CAD build for the part. Positions are in the model's coordinates, mm. A direction names the side the tool comes from. Give positions to 0.01 mm unless a question says otherwise; leave off trailing zeros. Write each loop counter-clockwise with the first axis right and the second up, starting at its lowest first coordinate (ties: lowest second). Pieces come first, ordered by that corner, then holes. Notation, with made-up numbers: (-31, 47) - (8, 47) arc R16 ccw to (8, 68) - close; hole circle Ø11 at (51, 38.25). An arc over 180 degrees is marked (long way). Write item = value, one per line. Start each with the question number.
```python
from build123d import *

# Parameters (mm, degrees)
ESQUISSE1_R             = 6
BOSS_EXTRU_1_DEPTH      = 10
ESQUISSE4_R             = 4.25
ESQUISSE4_R_2           = 3.25
ENL_V_MAT_EXTRU_1_DEPTH = 0.1


with BuildPart() as part:
    # Esquisse1 → Boss.-Extru.1 (new body)
    with BuildSketch(Plane(origin=(0, 0, 0), x_dir=(1, 0, 0), z_dir=(0, 1, 0))):
        with Locations(Location((0, 0, 0), (0, 0, 270))):
            Circle(ESQUISSE1_R)
    extrude(amount=-BOSS_EXTRU_1_DEPTH)

    # Esquisse3 → Révolution1 (revolve)
    with BuildSketch(Plane(origin=(0, 0, 0), x_dir=(0, 0, -1), z_dir=(1, 0, 0))):
        Polygon((0, 0), (0, 2), (5.25, 2), (6.85, 0), align=None)
    revolve(axis=Axis((0, 0, 0), (0, 1, 0)))

    # Esquisse4 → Enlèv. mat.-Extru.1 (cut)
    with BuildSketch(Plane(origin=(0, 2, 0), x_dir=(1, 0, 0), z_dir=(0, 1, 0))):
        with Locations(Location((0, 0, 0), (0, 0, 270))):
            Circle(ESQUISSE4_R)
        with Locations(Location((0, 0, 0), (0, 0, 270))):
            Circle(ESQUISSE4_R_2, mode=Mode.SUBTRACT)
    extrude(amount=-ENL_V_MAT_EXTRU_1_DEPTH, mode=Mode.SUBTRACT)


solid = part.part
```
1. Pin check, flat tips, straight feed: pin 1 Ø2 at (y, z) = (1, -4) entering from +X; pin 2 Ø1.5 at (x, y) = (-5, -4.5) entering from -Z; pin 3 Ø3 at (x, y) = (3, -2.5) entering from -Z. Stop position of each tip, or through.
2. Cut at C-C (y = -8.25). Give the cut face in (x, z).
3. Cut at B-B (x = 0). Give the cut face in (y, z).
4. Wall check: line 1 along X through (y, z) = (1.95, 0); line 2 along Y through (x, z) = (3.75, 1); line 3 along Z through (x, y) = (1, -8). Give the ranges that are in metal, low to high.
5. Tool access for faces 1 (the flat face through (4, 2, 2)), 2 (the flat face through (5, 0, -4)): list every direction of +Z, -Z, +X, -X, +Y, -Y with a clear straight run to the whole face (end or side of a thin tool).
6. Cut at A-A (z = 0). Give the cut face in (x, y).
Output:
q1.pin_1 = 5.76
q1.pin_2 = -4.24
q1.pin_3 = -5.81
q2.outline = circle Ø12 at (0, 0)
q3.outline = (-10, -6) - (0, -6) - (0, -6.85) - (2, -5.25) - (2, -4.25) - (1.9, -4.25) - (1.9, -3.25) - (2, -3.25) - (2, 3.25) - (1.9, 3.25) - (1.9, 4.25) - (2, 4.25) - (2, 5.25) - (0, 6.85) - (0, 6) - (-10, 6) - close
q4.line_1 = -5.29 to -4.25, -3.25 to 3.25, 4.25 to 5.29
q4.line_2 = -10 to 1.9
q4.line_3 = -5.92 to 5.92
q5.face_1 = +Z, -Z, +X, -X, +Y
q5.face_2 = -Y
q6.outline = (-6.85, 0) - (-6, 0) - (-6, -10) - (6, -10) - (6, 0) - (6.85, 0) - (5.25, 2) - (4.25, 2) - (4.25, 1.9) - (3.25, 1.9) - (3.25, 2) - (-3.25, 2) - (-3.25, 1.9) - (-4.25, 1.9) - (-4.25, 2) - (-5.25, 2) - close
